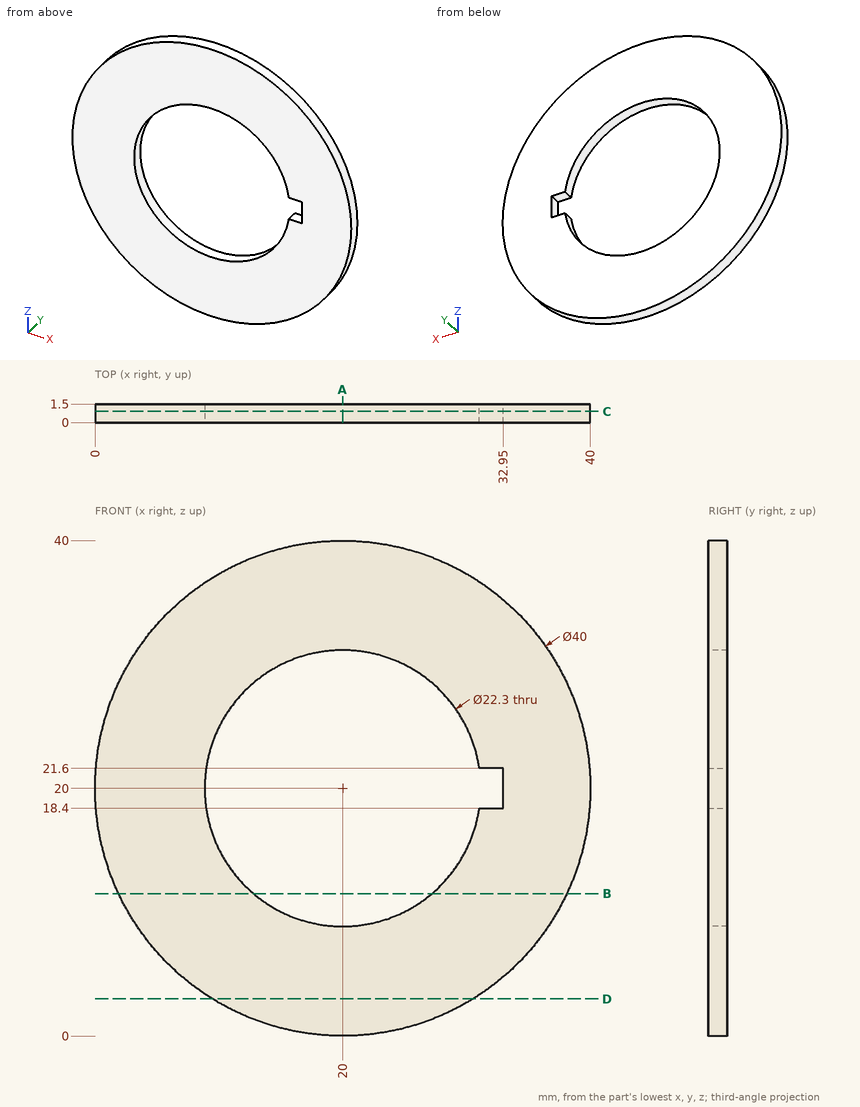
Check sheet for the drawn part. Datum: minimum x, y, z corner. Units: mm. Coordinates: 2 decimals unless noted, no trailing zeros. Order: outer loops, then holes, each group sorted by start corner. A loop starts at its lowest first (then second) coordinate and runs counter-clockwise, first axis right, second up. Notation, with made-up numbers: (14, 43) -> (22, 43) arc R25 cw to (22, 81) -> close; hole circle Ø4 at (64, 63). An arc over 180 degrees is marked (long way). Use a Markdown table: item, result. Add a question column.
1. Cross-section at D-D (z = 3). Enter the section's corners in (x, y).
2. Cross-section at C-C (y = 0.9). Enter the section's corners in (x, z).
3. Material ranges on L1, parallel to X at y = 0.9, z = 20; L2, parallel to Z at x = 20, y = 1.1; L3, parallel to X at y = 0.85, z = 13.5, recorded low to high.
4. Cross-section at A-A (x = 20). Enter the section's corners in (y, z), and give its area (4 significant figures).
5. Cross-section at B-B (z = 11.5). Enter the section's corners in (x, y), and give its area (3 significant figures).
Filled sheet:
| question | item | result |
|---|---|---|
| 1 | outline | (9.46, 0) -> (30.54, 0) -> (30.54, 1.5) -> (9.46, 1.5) -> close |
| 2 | outline | circle Ø40 at (20, 20); hole (31.03, 18.4) -> (32.95, 18.4) -> (32.95, 21.6) -> (31.03, 21.6) arc R11.15 ccw (long way) to start |
| 3 | L1 | 0 to 8.85, 32.95 to 40 |
| 3 | L2 | 0 to 8.85, 31.15 to 40 |
| 3 | L3 | 1.09 to 10.94, 29.06 to 38.91 |
| 4 | outline | (0, 0) -> (1.5, 0) -> (1.5, 8.85) -> (0, 8.85) -> close; (0, 31.15) -> (1.5, 31.15) -> (1.5, 40) -> (0, 40) -> close |
| 4 | area | 26.55 mm2 |
| 5 | outline | (1.9, 0) -> (12.78, 0) -> (12.78, 1.5) -> (1.9, 1.5) -> close; (27.22, 0) -> (38.1, 0) -> (38.1, 1.5) -> (27.22, 1.5) -> close |
| 5 | area | 32.7 mm2 |
